Input: dimensioned drawing with shaded views. Units: mm. Origin: part minimum x, y, z. A direction names the side the tool comes from. Give positions to 0.01 mm unless a question says otherwise; leave off trailing zeros. Write each loop counter-clockwise with the first axis right and the second up, starting at its lowest first coordinate (ties: lowest second). Pieces come first, ordered by that corner, then holes. Notation, with made-up numbers: (65, 3.5) -> (81, 3.5) arc R19 cw to (81, 32.5) -> close; hole circle Ø7 at (27, 32). An arc over 180 degrees is marked (long way). Answer as a JSON object with one key per item and string values. Group by question number.
(1) Material intervals for probe 1 along Y at (x, z) = (12.5, 11); probe 2 along Y at (x, z) = (3.25, 26.35); probe 3 along X at (y, z) = (5.5, 22), sorted ascending.
(2) Contact query for flat-ended pins moving along their axis: pin 1 Ø6 at (y, z) = (6.37, 26.35) entering from +X; pin 2 Ø10 at (x, y) = (14, 8) entering from +Z; pin 3 Ø6 at (x, z) = (12.35, 6.37) entering from -Y; pin 4 Ø3 at (y, z) = (17, 10) entering from -X. Output: stop coordinate, or through.
(3) Section query C-C on z = 6.37. Output: boundary loops of the cut face in (x, y).
(4) Draft query along Y for the marked faces 1, 2 and 3. Return one class per face: +Y half, -Y half, draft (parallel to the pull), parting line (faces both ways), or undercut.
(5) Section query D-D on y = 11.5. Output: boundary loops of the cut face in (x, z), plus the area to 3 significant figures.
(6) Set-up query: the marked faces 4, 5, 6 and 7. Return all of +Z, -Z, +X, -X, +Y, -Y with unobstructed straight access to the full face (end or side cutting, diameter ignored); none if empty.
(7) Section query B-B on y = 6.37. Output: boundary loops of the cut face in (x, z), plus the area to 3 significant figures.
(8) Section query A-A on x = 12.35. Output: boundary loops of the cut face in (y, z), plus the area to 3 significant figures.
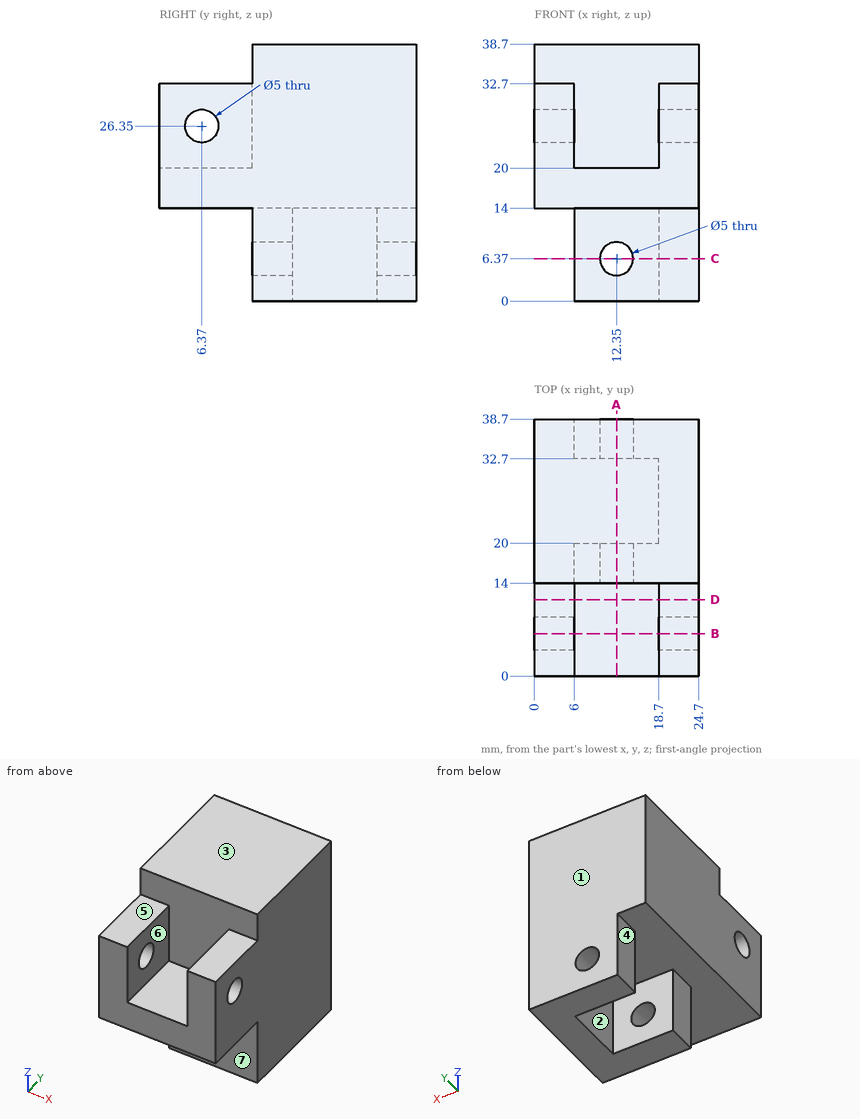
Answer list:
{
 "1": {"probe 1": "14 to 20, 32.7 to 38.7", "probe 2": "0 to 3.87, 8.87 to 38.7", "probe 3": "0 to 6, 18.7 to 24.7"},
 "2": {"pin 1": "x = 24.7", "pin 2": "z = 32.7", "pin 3": "y = 14", "pin 4": "x = 6"},
 "3": {"outline": "(6, 14) -> (9.85, 14) -> (9.85, 20) -> (6, 20) -> close; (6, 32.7) -> (9.85, 32.7) -> (9.85, 38.7) -> (6, 38.7) -> close; (14.85, 14) -> (24.7, 14) -> (24.7, 38.7) -> (14.85, 38.7) -> (14.85, 32.7) -> (18.7, 32.7) -> (18.7, 20) -> (14.85, 20) -> close"},
 "4": {"face 1": "+Y half", "face 2": "undercut", "face 3": "draft"},
 "5": {"outline": "(0, 14) -> (24.7, 14) -> (24.7, 32.7) -> (18.7, 32.7) -> (18.7, 20) -> (6, 20) -> (6, 32.7) -> (0, 32.7) -> close", "area": "301 mm2"},
 "6": {"face 4": "-Z, -X, +Y, -Y", "face 5": "+Z, +X, -X, -Y", "face 6": "+Z, -Y", "face 7": "-Z, +X, -X, -Y"},
 "7": {"outline": "(0, 14) -> (24.7, 14) -> (24.7, 23.85) -> (18.7, 23.85) -> (18.7, 20) -> (6, 20) -> (6, 23.85) -> (0, 23.85) -> close; (0, 28.85) -> (6, 28.85) -> (6, 32.7) -> (0, 32.7) -> close; (18.7, 28.85) -> (24.7, 28.85) -> (24.7, 32.7) -> (18.7, 32.7) -> close", "area": "241 mm2"},
 "8": {"outline": "(0, 14) -> (14, 14) -> (14, 8.87) -> (20, 8.87) -> (20, 14) -> (32.7, 14) -> (32.7, 8.87) -> (38.7, 8.87) -> (38.7, 38.7) -> (14, 38.7) -> (14, 20) -> (0, 20) -> close; (14, 0) -> (20, 0) -> (20, 3.87) -> (14, 3.87) -> close; (32.7, 0) -> (38.7, 0) -> (38.7, 3.87) -> (32.7, 3.87) -> close", "area": "802 mm2"}
}
